Source: three-view drawing plus pictorial views. Frame: mm from the lowest corner of the part. A direction names the side the tool comes from. Give positions to 0.01 mm unless a question says otherwise; leave off trailing zeros. Loops run counter-clockwise (first coordinate to the right, second up) from the corner with the lowest first, then second, coordinate; pieces in that order, holes last. Notation, with made-up numbers: (-33.75, 34) - (16.25, 34) arc R17 cw to (16.25, 64) - close; hole circle Ø9 at (20.5, 19). An arc over 180 degrees is marked (long way). Answer as a JSON object with one key per item and string values.
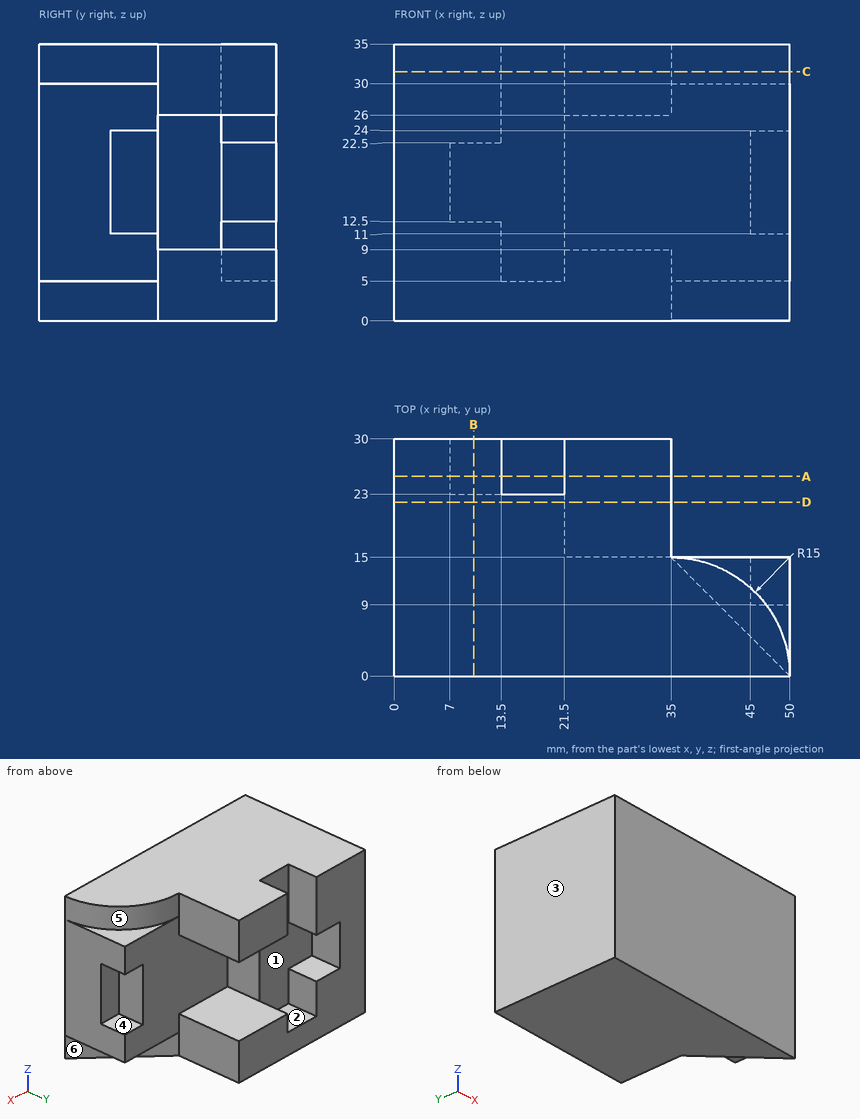
Item 1: Cut plane D-D (y = 22). Return loops of the section in (x, z).
Geometry check:
{"outline": "(0, 0) - (35, 0) - (35, 9) - (21.5, 9) - (21.5, 26) - (35, 26) - (35, 35) - (0, 35) - close"}
Item 2: Cut plane B-B (x = 10). Return loops of the section in (y, z), then the cut area to 3 significant figures.
Geometry check:
{"outline": "(0, 0) - (30, 0) - (30, 12.5) - (23, 12.5) - (23, 22.5) - (30, 22.5) - (30, 35) - (0, 35) - close", "area": "980 mm2"}
Item 3: Mould query, pull axis Z, two halves, no side actions, for the marked faces 1, 2 and 3. Classes: released by +Z, released by -Z, zero draft, split by the parting line, or undercut.
Geometry check:
{"face 1": "undercut", "face 2": "released by +Z", "face 3": "zero draft"}
Item 4: Cut plane C-C (z = 31.5). Return loops of the section in (x, y).
Geometry check:
{"outline": "(0, 0) - (50, 0) arc R15 ccw to (35, 15) - (35, 30) - (21.5, 30) - (21.5, 23) - (13.5, 23) - (13.5, 30) - (0, 30) - close"}
Item 5: Material intervals for line 1 (X direction, y = 28.5, z = 8); line 2 (Z direction, x = 27.5, y = 17); line 3 (Y direction, x = 29, z = 9.5), sorted ascending. Write a range as [from, to].
Geometry check:
{"line 1": "x = [0, 13.5], [21.5, 35]", "line 2": "z = [0, 9], [26, 35]", "line 3": "y = [0, 15]"}
Item 6: Cut plane A-A (y = 25.25). Return loops of the section in (x, z).
Geometry check:
{"outline": "(0, 0) - (35, 0) - (35, 9) - (21.5, 9) - (21.5, 5) - (13.5, 5) - (13.5, 12.5) - (7, 12.5) - (7, 22.5) - (13.5, 22.5) - (13.5, 35) - (0, 35) - close; (21.5, 26) - (35, 26) - (35, 35) - (21.5, 35) - close"}
Item 7: Access query for the marked faces 4, 5 and 6. Directions: +Z, -Z, +X, -X, +Y, -Y. A direction counts if a zero-diameter tool reaches every point of the face in a straight line with its end or side. Return the directions, or none.
Geometry check:
{"face 4": "+X, +Y", "face 5": "+Z, +X, +Y", "face 6": "-Z, +X, +Y"}
Item 8: Contact query for flat-ended pins moving along their axis: P1, Ø2, axis at y = 26, z = 30.5, coming from the -X side; P2, Ø1.8, axis at y = 12, z = 20, coming from the +X side; P3, Ø3.5, axis at x = 16.5, y = 28, coming from the +Z side; P4, Ø5.5, axis at y = 25, z = 19.5, coming from the +X side. Output: stop coordinate, or through.
Geometry check:
{"P1": "stops at x = 0", "P2": "stops at x = 45", "P3": "stops at z = 5", "P4": "stops at x = 21.5"}
